Autodesk Inventor part; units mm, degrees
ref_plane "Work Plane1" through (40, -59.8973, -11.9951) normal (0, 0, -1) x (0, 1, 0)
ref_plane "YZ Plane" through (0, 0, 0) normal (1, 0, 0) x (0, 1, 0)
ref_plane "XZ Plane" through (0, 0, 0) normal (0, 1, 0) x (-1, 0, 0)
ref_plane "Work Plane1" through (40, -59.8973, -11.9951) normal (0, 0, -1) x (0, 1, 0)
sketch "Sketch1" plane through (0, 0, 0) normal (0, 0, 1) x (1, 0, 0)
  line L0 (2.5, -40.193) -> (20, -40.193)
  line L1 (20, -31.5948) -> (20, -40.193)
  line L2 (20, -31.5948) -> (2.5, -31.5948)
  line L3 (2.5, -31.5948) -> (2.5, -19.0948)
  line L4 (2.5, -19.0948) -> (20, -19.0948)
  line L5 (20, -10.4966) -> (20, -19.0948)
  line L6 (20, -10.4966) -> (2.5, -10.4966)
  line L7 (2.5, -10.4966) -> (2.5, 2.0034)
  line L8 (2.5, 2.0034) -> (20, 2.0034)
  line L9 (20, 12.0034) -> (20, 2.0034)
  line L10 (-7.708, 12.0034) -> (20, 12.0034)
  line L11 (-7.708, -62.693) -> (-7.708, 12.0034)
  line L12 (-7.708, -62.693) -> (20, -62.693)
  line L13 (20, -52.693) -> (20, -62.693)
  line L14 (20, -52.693) -> (2.5, -52.693)
  line L15 (2.5, -52.693) -> (2.5, -40.193)
  line L16 (57.5, -10.4966) -> (40, -10.4966)
  line L17 (40, -19.0948) -> (40, -10.4966)
  line L18 (40, -19.0948) -> (57.5, -19.0948)
  line L19 (57.5, -19.0948) -> (57.5, -31.5948)
  line L20 (57.5, -31.5948) -> (40, -31.5948)
  line L21 (40, -40.193) -> (40, -31.5948)
  line L22 (40, -40.193) -> (57.5, -40.193)
  line L23 (57.5, -40.193) -> (57.5, -52.693)
  line L24 (57.5, -52.693) -> (40, -52.693)
  line L25 (40, -62.693) -> (40, -52.693)
  line L26 (67.708, -62.693) -> (40, -62.693)
  line L27 (67.708, 12.0034) -> (67.708, -62.693)
  line L28 (67.708, 12.0034) -> (40, 12.0034)
  line L29 (40, 2.0034) -> (40, 12.0034)
  line L30 (40, 2.0034) -> (57.5, 2.0034)
  line L31 (57.5, 2.0034) -> (57.5, -10.4966)
  line L32 (20, 12.0034) -> (40, 12.0034)
  line L33 (40, -187.9966) -> (20, -187.9966)
  line L34 (57.5, -62.693) -> (57.5, -75.193)
  line L35 (57.5, -75.193) -> (40, -75.193)
  line L36 (40, -75.193) -> (40, -187.9966)
  line L37 (2.5, -62.693) -> (2.5, -75.193)
  line L38 (2.5, -75.193) -> (20, -75.193)
  line L39 (20, -75.193) -> (20, -187.9966)
  point P0 (0, 0)
  dimension "d0" = 200
  dimension "d1" = 17.5
  dimension "d2" = 17.5
  dimension "d3" = 12.5
extrude "Extrusion1" add sketch "Sketch1" against normal up to surface (11.9951 mm away) contours L0 L1 L2 L3 L4 L5 L6 L7 L8 L9 L32 L29 L30 L31 L16 L17 L18 L19 L20 L21 L22 L23 L24 L25 L26 L34 L35 L36 L33 L39 L38 L37 L12 L13 L14 L15
sketch "Sketch2" plane through (2.5, -75.193, 0) normal (0, -1, 0) x (1, 0, 0)
  line L0 (0, -11.9951) -> (17.5, -11.9951)
  line L1 (17.5, 0) -> (17.5, -11.9951)
  line L2 (0, 0) -> (17.5, 0)
  line L3 (0, 0) -> (0, -11.9951)
  line L4 (0, 0) -> (17.5, 0)
  line L5 (17.5, 0) -> (17.5, -11.9951)
  line L6 (0, 0) -> (17.5, -11.9951)
  circle A0 centre (10, -6.6174) radius 3.3205
  point P0 (-2.5, 0)
sketch "Sketch3" plane through (2.5, 2.0034, 0) normal (0, 1, 0) x (1, 0, 0)
  circle A0 centre (8.75, 5.9976) radius 2.5
  circle A1 centre (8.75, 5.9976) radius 2.5
  line L0 (0, 0) -> (17.5, 0)
  line L1 (17.5, 0) -> (17.5, 11.9951) construction
  line L2 (0, 0) -> (17.5, 11.9951) construction
  line L3 (17.5, 11.9951) -> (0, 11.9951) construction
  line L4 (0, 11.9951) -> (17.5, 0) construction
  line L5 (37.5, 0) -> (37.5, 11.9951) construction
  line L6 (37.5, 11.9951) -> (55, 11.9951) construction
  line L7 (37.5, 0) -> (55, 11.9951) construction
  line L8 (55, 11.9951) -> (37.5, 11.9951) construction
  line L9 (37.5, 11.9951) -> (55, 0) construction
  circle A2 centre (46.25, 5.9976) radius 2.5
  point P0 (-2.5, 0)
  dimension "d7" = 5
extrude "Extrusion2" cut sketch "Sketch3" against normal blind 86.2
properties part number "Center"
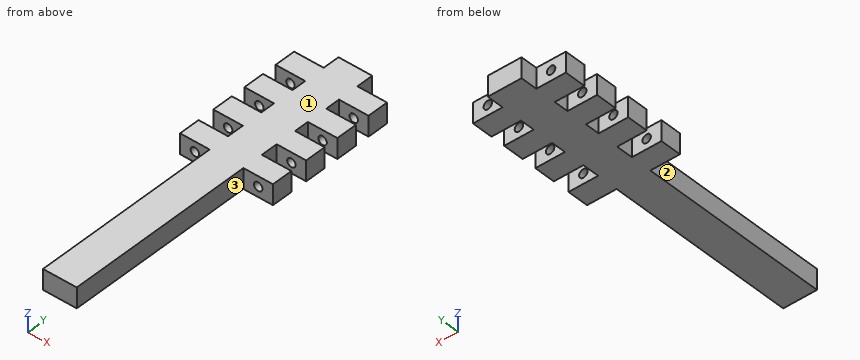
The model under review builds one solid part; all positions refer to its coordinate system, in mm. Face numbers are marked on the shaded views. A direction names the side the tool comes from. Coordinates: 2 decimals unless noted, no trailing zeros. Loops run counter-clockwise (first coordinate to the right, second up) from the corner with the lowest first, then second, coordinate; pieces in that order, holes last.
(1) Consider section C-C, the plane y = -72. Give the boundary of the cut face in (x, z), plus the area to 3 significant figures.
Determined:
outline: (2.5, -12) - (57.5, -12) - (57.5, 0) - (2.5, 0) - close; hole circle Ø5 at (11.25, -6); hole circle Ø5 at (48.75, -6)
area: 620 mm2
(2) Consider section A-A, the plane x = 43. Give the boundary of the cut face in (y, z), plus the area to 3 significant figures.
Determined:
outline: (-75.19, -12) - (-62.69, -12) - (-62.69, 0) - (-75.19, 0) - close; (-52.69, -12) - (-40.19, -12) - (-40.19, 0) - (-52.69, 0) - close; (-31.59, -12) - (-19.09, -12) - (-19.09, 0) - (-31.59, 0) - close; (-10.5, -12) - (2, -12) - (2, 0) - (-10.5, 0) - close
area: 600 mm2
(3) Insertion check: P1, Ø6, axis at x = 15.5, z = -3, coming from the -Y side; P2, Ø7, axis at y = -35.5, z = -4, coming from the +X side; P3, Ø3, axis at x = 48.75, z = -6, coming from the +Y side; P4, Ø6.5, axis at x = 48.75, z = -6, coming from the +Y side. Each pin has a flat end and moves straight along its axis. Give the tip position at first contact, or say it passes through.
Determined:
P1: stops at y = -75.19
P2: stops at x = 40
P3: passes through
P4: stops at y = 2
(4) Consider section D-D, the plane y = -139. Give the boundary of the cut face in (x, z), plus the area to 3 significant figures.
Determined:
outline: (20, -12) - (40, -12) - (40, 0) - (20, 0) - close
area: 240 mm2
(5) Wall thickness on L1, parallel to Y at x = 14.5, z = -9; L2, parallel to Z at x = 11.25, y = -4.75; L3, parallel to X at y = -17.5, z = -0.25: over which ranges is each line inside the solid? List them lowest first.
Determined:
L1: y = -75.19 to -62.69, -52.69 to -40.19, -31.59 to -19.09, -10.5 to 2
L2: z = -12 to -8.5, -3.5 to 0
L3: x = 20 to 40
(6) Tool access review of the marked faces 1, 2 and 3: name each direction out of +Z, -Z, +X, -X, +Y, -Y from which nothing blocks a thin tool from reaching the whole face with its end or side.
Determined:
face 1: +Z, +X, -X, +Y, -Y
face 2: +Z, -Z, -X, -Y
face 3: +Z, -Z, +X, -Y
(7) Consider section B-B, the plane x = 11.25. Give the number of separate pieces and of enclosed holes in the cut face, plus the area to 3 significant figures.
Determined:
separate pieces: 8
enclosed holes: 0
area: 350 mm2
